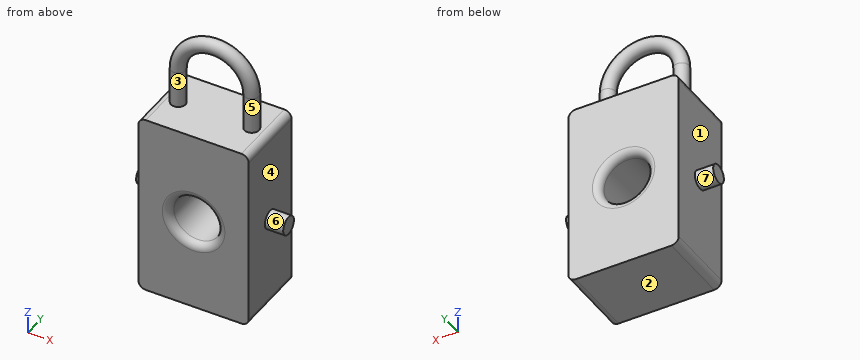
from build123d import *

# Parameters (mm, degrees)
F0_W     = 150
F0_H     = 100
F1_DEPTH = 250
F2_R     = 32.5
F3_DEPTH = 100.001
F4_R     = 10
F5_R     = 12.5
F6_DEPTH = 25
F7_R     = 10


# Not quite as in the source:
# - a pattern or mirror of a feature is missing from the dataset's text; its kind, count and spacing are read off the source's solid


with BuildPart() as f1:
    # F0 (on Top) → F1 (new body)
    with BuildSketch(Plane.XY):
        Rectangle(F0_W, F0_H)
    extrude(amount=F1_DEPTH)

    # F2 (on face) → F3 (cut, through all)
    with BuildSketch(Plane(origin=(0, 50, 0), x_dir=(-1, 0, 0), z_dir=(0, 1, 0))):
        with Locations((0, 125)):
            Circle(F2_R)
    extrude(amount=-F3_DEPTH, mode=Mode.SUBTRACT)

    # F4
    f4_edges = [f1.edges().sort_by_distance(p)[0] for p in [
        (-75, 0, 250),
        (75, 0, 250),
        (75, 0, 0),
        (-75, 0, 0),
        (32.5, -50, 125),
        (32.5, 50, 125),
    ]]
    fillet(f4_edges, radius=F4_R)

    # F5 (on face) → F6 (join)
    with BuildSketch(Plane(origin=(-75, 0, 0), x_dir=(0, -1, 0), z_dir=(-1, 0, 0))):
        with Locations((0, 125)):
            Circle(F5_R)
    f6 = extrude(amount=F6_DEPTH)

    # F6_copies: F6 across plane
    add(f6.mirror(Plane(origin=(0, 0, 0), x_dir=(0, 0, 1), z_dir=(1, 0, 0))))

    # F9: sweep along a path in F8
    with BuildLine(Plane.XZ) as f9_path:
        Line((-50, 250), (-50, 300))
        ThreePointArc((-50, 300), (0, 350), (50, 300))
        Line((50, 300), (50, 250))
    # F7 (on face) → F9 (sweep)
    with BuildSketch(Plane.XY.offset(250)):
        with Locations((50, 0)):
            Circle(F7_R)
    sweep(path=f9_path.line)


solid = f1.part
Can you work these out from the model? Positions are in its coordinate system, mm. Face numbers are marked on the shaded views. A direction names the side the tool comes from. Round coordinates to 2 decimals unless told otherwise and drop trailing zeros. Order: outer loops, then holes, each group sorted by start corner. A loop starts at its lowest first (then second) coordinate and runs counter-clockwise, first axis right, second up. Notation, with made-up numbers: M 52,-19.5 L 63,-19.5 A27 ccw 63,-1.5 Z; hole C 57.25,42.25 d11. An arc over 180 degrees is marked long. Use a Markdown table: item, result.
1) Imagine slicing it at C-C (y = 0). List the corners of the cut face in (x, z) for me.
Geometry says:
| item | result |
|---|---|
| outline | M -100,112.5 L -75,112.5 L -75,10 A10 ccw -65,0 L 65,0 A10 ccw 75,10 L 75,112.5 L 100,112.5 L 100,137.5 L 75,137.5 L 75,240 A10 ccw 65,250 L 60,250 L 60,300 A60 ccw -60,300 L -60,250 L -65,250 A10 ccw -75,240 L -75,137.5 L -100,137.5 Z; hole M -40,250 L 40,250 L 40,300 A40 ccw -40,300 Z; hole C 0,125 d65 |
2) Imagine slicing it at A-A (x = 0). List the corners of the cut face in (y, z) for me, then the cut area to 3 significant figures.
Geometry says:
| item | result |
|---|---|
| outline | M -50,0 L 50,0 L 50,82.5 A10 ccw 40,92.5 L -40,92.5 A10 ccw -50,82.5 Z; M -50,167.5 A10 ccw -40,157.5 L 40,157.5 A10 ccw 50,167.5 L 50,250 L -50,250 Z; C 0,350 d20 |
| area | 18,700 mm² |
3) If we mould it in two halves opening along X, with no side actions, what happens to the marked faces 1, 2, 3 and 4? For each: +X half, -X half, draft (parallel to the pull), parting line (faces both ways), or undercut.
Geometry says:
| item | result |
|---|---|
| face 1 | -X half |
| face 2 | draft |
| face 3 | undercut |
| face 4 | +X half |
4) Imagine slicing it at D-D (z = 277). List the corners of the cut face in (x, y) for me.
Geometry says:
| item | result |
|---|---|
| outline | C -50,0 d20; C 50,0 d20 |
5) I'm going to push flat-ended pins straight in: P1, Ø12, axis at y = 23, z = 128.5, coming from the -X side; P2, Ø4, axis at x = -59.5, y = -28, coming from the +Z side; P3, Ø4, axis at x = -71.5, y = 14, coming from the -Z side. Where does each tip first touch, or does it pass through?
Geometry says:
| item | result |
|---|---|
| P1 | stops at x = -75 |
| P2 | stops at z = 250 |
| P3 | stops at z = 1.07 |
6) Imagine slicing it at B-B (y = 18.5). List the corners of the cut face in (x, z) for me.
Geometry says:
| item | result |
|---|---|
| outline | M -75,10 A10 ccw -65,0 L 65,0 A10 ccw 75,10 L 75,240 A10 ccw 65,250 L -65,250 A10 ccw -75,240 Z; hole C 0,125 d65 |
7) If I drill on line 1 along Z through (x, y) = (0, -5); line 2 along Z through (x, y) = (0, 7); line 3 along X through (y, z) = (-26, 148), over which ranges is the centre line in solid material (lowest first)?
Geometry says:
| item | result |
|---|---|
| line 1 | z = 0 to 92.5, 157.5 to 250, 341.34 to 358.66 |
| line 2 | z = 0 to 92.5, 157.5 to 250, 342.86 to 357.14 |
| line 3 | x = -75 to -22.96, 22.96 to 75 |
8) On a 3-axis mill with a long thin cutter (end or side, diameter ignored), from which of +Z, -Z, +X, -X, +Y, -Y can I reach the whole of each face in a straight line? I mean the marked faces 5, 6 and 7. Say none if no direction works.
Geometry says:
| item | result |
|---|---|
| face 5 | none |
| face 6 | +X |
| face 7 | -X |
